The model under review builds one solid part; all positions refer to its coordinate system, in mm. A direction names the side the tool comes from. Coordinates: 2 decimals unless noted, no trailing zeros. Write each loop counter-clockwise with the first axis right and the second up, starting at its lowest first coordinate (ties: lowest second). Pieces come first, ordered by that corner, then holes. Notation, with made-up numbers: (87, -10.5) - (136, -10.5) arc R10 cw to (136, 5.5) - close; hole circle Ø6 at (3, 77). An arc over 180 degrees is marked (long way). Answer as CSV lines item,"result". Start each with the question number.
```python
from build123d import *

# Parameters (mm, degrees)
SKETCH001_R        = 4.007612
PAD_DEPTH          = 8.5
POLARPATTERN_COUNT = 12


with BuildPart() as part:
    # Sketch → Revolution (revolve)
    with BuildSketch(Plane.XY):
        with BuildLine():
            Line((55.236058, 58.551815), (52.99765, 56.810364))
            Line((52.99765, 56.810364), (52.99765, 38.823368))
            Line((52.99765, 38.823368), (60.170532, 38.823368))
            Line((60.170532, 38.823368), (60.170532, 30.492123))
            Line((60.170532, 30.492123), (53.057545, 30.492123))
            Line((53.057545, 30.492123), (53.057545, 28.663067))
            Line((53.057545, 28.663067), (50.618809, 28.663067))
            Line((50.618809, 28.663067), (50.618809, 0))
            Line((50.618809, 0), (0, 0))
            Line((0, 0), (0, 58.55183))
            Line((0, 113.787847), (0, 58.55183))
            ThreePointArc((55.236058, 58.551815), (40.402433, 98.954241), (0, 113.787847))
        make_face()
    revolve(axis=Axis((0, 0, 0), (0, 1, 0)))

    # Sketch001 → Pad (new body)
    with BuildSketch(Plane.XZ.offset(-30.5)):
        with Locations((0, 59.889767)):
            Circle(SKETCH001_R)
    pad = extrude(amount=-PAD_DEPTH)

    # PolarPattern: Pad ×12 about axis
    polarpattern_axis = Axis((0, 30.5, 0), (0, -1, 0))
    for i in range(1, POLARPATTERN_COUNT):
        add(pad.rotate(polarpattern_axis, i * 360 / POLARPATTERN_COUNT))


solid = part.part
```
(1) For pin 1 (4 mm diameter, centred on x = -9.5, z = 50.5, fed in from +Y); pin 2 (6.5 mm diameter, centred on x = -52.5, z = -29, fed in from -Y); pin 3 (2.5 mm diameter, centred on x = 59, z = -1, fed in from +Y); pin 4 (10 mm diameter, centred on x = -3, z = -10, fed in from -Y), all flat-tipped, find the tip position at first contact; note any pin that passes through.
(2) For faces 1 (the flat face through (-53, 30.5, 31)), 2 (the flat face through (-52, 39, -30)), 3 (the flat face through (31, 30.5, 53)), 4 (the flat face through (-31, 30.5, -53)), list the 3-axis set-ups (+Z, -Z, +X, -X, +Y, -Y) from which the entire face can be reached by the end or side of a thin tool; tool diameter is ignored.
(3) The part is to be moulded in two halves that separate along Z. For faces 5 (the flat face through (46.915, 28.663, 19.403)), 6 (the cylindrical face through (-55.05, 34.69, -32.38)), say which applies: released by +Z, released by -Z, zero draft, split by the parting line, or undercut.
(4) Add section A-A on y = 16. Give the boundary of the cut face in (x, z), then the cut area to 3 significant figures.
(5) Wall thickness on line 1 (Y direction, x = -29, z = 47.5); line 2 (Y direction, x = 53.5, z = -32); line 3 (X direction, y = 52, z = 4.5): over which ranges is each line inside the solid? List them lowest first.
Reported:
1,pin 1,"y = 86.83"
1,pin 2,"y = 30.49"
1,pin 3,"y = 39"
1,pin 4,"y = 0"
2,face 1,"+Z, -X, -Y"
2,face 2,"-Z, -X, +Y"
2,face 3,"+Z, +X, -Y"
2,face 4,"-Z, -X, -Y"
3,face 5,"zero draft"
3,face 6,"undercut"
4,outline,"circle Ø101.24 at (0, 0)"
4,area,"8,050 mm²"
5,line 1,"30.49 to 38.82"
5,line 2,"30.5 to 39"
5,line 3,"-52.81 to 52.81"
